The drawing under review shows one solid part. Ordinate dimensions are in mm from its lowest x, y, z. Round coordinates to 2 decimals unless told otherwise and drop trailing zeros. Order: outer loops, then holes, each group sorted by start corner. A loop starts at its lowest first (then second) coordinate and runs counter-clockwise, first axis right, second up. Notation, with made-up numbers: (80, -37.5) -> (93, -37.5) arc R7 cw to (93, -28.5) -> close; hole circle Ø7 at (10.5, -26). An arc over 180 degrees is marked (long way). Put each result on its own line as item: value. Start each with the question number.
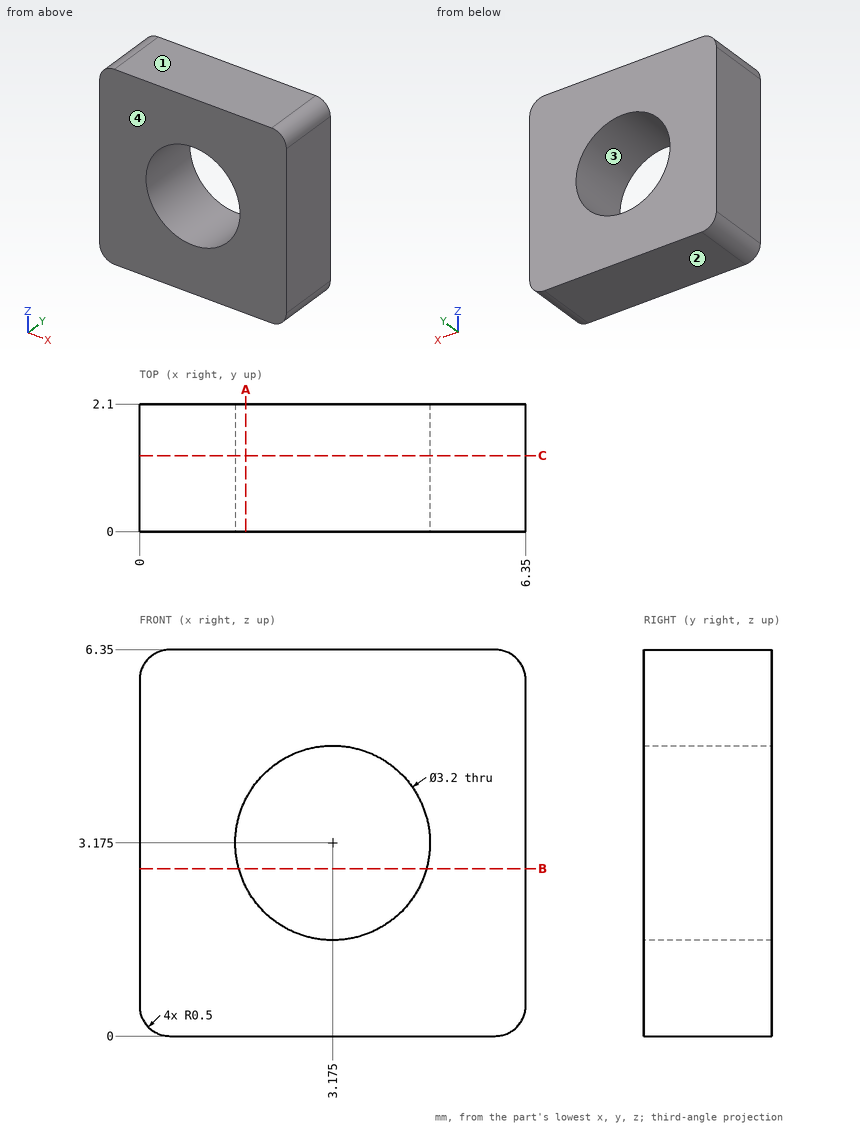
Item 1: Insertion check: pin 1 Ø3.5 at (x, z) = (3.175, 3.175) entering from -Y. The pin has a flat end and moves straight along its axis. Give the tip position at first contact, or say it passes through.
Item 2: Consider section C-C, the plane y = 1.25. Write out the cut boundary in (x, z) (3 decimals), plus the area to 3 significant figures.
Item 3: For L1, parallel to Z at x = 3.25, y = 0.1; L2, parallel to Z at x = 3.5, y = 0.4; L3, parallel to X at y = 1.6, z = 4.5, list the stretches that pass through material, from the lowest coordinate up.
Item 4: Mouldability with a two-part tool opening along Z and no side actions: class the marked faces 1, 2, 3 and 4 as +Z half, -Z half, draft (parallel to the pull), parting line (faces both ways), or undercut.
Item 5: Consider section A-A, the plane x = 1.75. Write out the cut boundary in (y, z), plus the area to 3 significant figures.
Item 6: Consider section B-B, the plane z = 2.75. Write out the cut boundary in (x, y), plus the area to 3 significant figures.
Evaluation:
1. pin 1: stops at y = 0
2. outline: (0, 0.5) arc R0.5 ccw to (0.5, 0) -> (5.85, 0) arc R0.5 ccw to (6.35, 0.5) -> (6.35, 5.85) arc R0.5 ccw to (5.85, 6.35) -> (0.5, 6.35) arc R0.5 ccw to (0, 5.85) -> close; hole circle Ø3.2 at (3.175, 3.175)
2. area: 32.1 mm^2
3. L1: z = 0 to 1.58, 4.77 to 6.35
3. L2: z = 0 to 1.61, 4.74 to 6.35
3. L3: x = 0 to 2.28, 4.07 to 6.35
4. face 1: +Z half
4. face 2: -Z half
4. face 3: undercut
4. face 4: draft
5. outline: (0, 0) -> (2.1, 0) -> (2.1, 2.45) -> (0, 2.45) -> close; (0, 3.9) -> (2.1, 3.9) -> (2.1, 6.35) -> (0, 6.35) -> close
5. area: 10.3 mm^2
6. outline: (0, 0) -> (1.63, 0) -> (1.63, 2.1) -> (0, 2.1) -> close; (4.72, 0) -> (6.35, 0) -> (6.35, 2.1) -> (4.72, 2.1) -> close
6. area: 6.86 mm^2
